Job drawing, mm, ordinate dimensions from the low corner. One solid piece. Round coordinates to 2 decimals unless told otherwise and drop trailing zeros. Loops run counter-clockwise (first coordinate to the right, second up) from the corner with the lowest first, then second, coordinate; pieces in that order, holes last. Notation, with made-up numbers: (82, 31) - (121, 31) arc R29 cw to (121, 56) - close; hole circle Ø5 at (75.25, 10). An arc over 180 degrees is marked (long way). One line per question, with ' | ' between items. Start each with the question number.
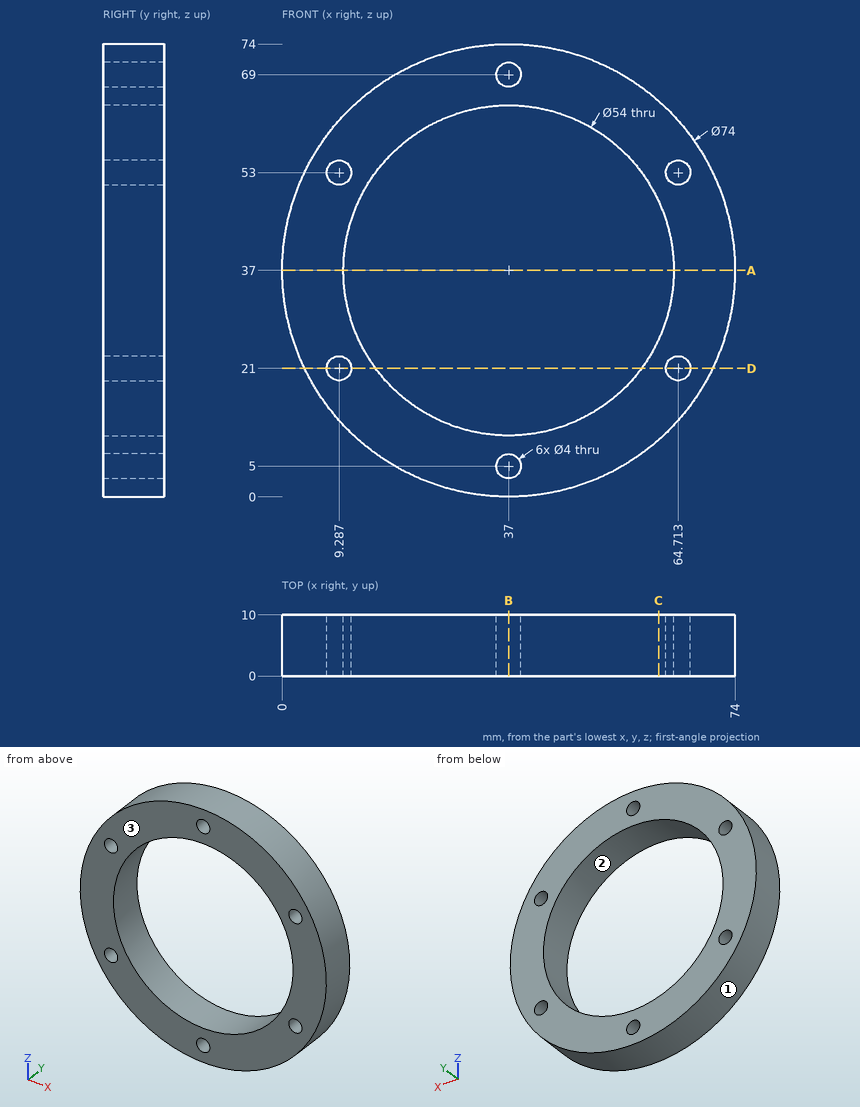
1) Wall check: line 1 (X direction, y = 7.5, z = 21); line 2 (X direction, y = 1.75, z = 19.5) (1 decimal); line 3 (X direction, y = 6, z = 37). Give the ranges that are in metal, low to high. Write a range as [from, to].
2) Saw through at B-B on x = 37. Write the cut outline in (y, z).
3) Saw through at A-A on z = 37. Write the cut outline in (x, y), and give its area (3 significant figures).
4) Saw through at D-D on z = 21. Write the cut outline in (x, y), and give its area (3 significant figures).
5) Drop flat-ended pins along their axis: pin 1 (3 mm diameter, centred on x = 8, y = 6.5, fed in from +Z); pin 2 (6 mm diameter, centred on y = 3, z = 65.5, fed in from -X); pin 3 (2 mm diameter, centred on y = 6, z = 19, fed in from -X). Give the stop position or say it passes through.
6) Two-plate mould, pull along X, no slides. Class the marked faces 1, 2 and 3: +X half, -X half, draft (parallel to the pull), parting line (faces both ways), or undercut.
7) Saw through at C-C on x = 61.5. Write the cut outline in (y, z), and give its area (3 significant figures).
Answer key:
1) line 1: [3.64, 7.29], [11.29, 15.25], [58.75, 62.71], [66.71, 70.36] | line 2: [4.4, 8], [10.6, 16.4], [57.6, 63.4], [66, 69.6] | line 3: [0, 10], [64, 74]
2) outline: (0, 0) - (10, 0) - (10, 3) - (0, 3) - close; (0, 7) - (10, 7) - (10, 10) - (0, 10) - close; (0, 64) - (10, 64) - (10, 67) - (0, 67) - close; (0, 71) - (10, 71) - (10, 74) - (0, 74) - close
3) outline: (0, 0) - (10, 0) - (10, 10) - (0, 10) - close; (64, 0) - (74, 0) - (74, 10) - (64, 10) - close | area: 200 mm²
4) outline: (3.64, 0) - (7.29, 0) - (7.29, 10) - (3.64, 10) - close; (11.29, 0) - (15.25, 0) - (15.25, 10) - (11.29, 10) - close; (58.75, 0) - (62.71, 0) - (62.71, 10) - (58.75, 10) - close; (66.71, 0) - (70.36, 0) - (70.36, 10) - (66.71, 10) - close | area: 152 mm²
5) pin 1: z = 61.75 | pin 2: x = 10.19 | pin 3: x = 4.14
6) face 1: parting line | face 2: undercut | face 3: draft
7) outline: (0, 9.27) - (10, 9.27) - (10, 25.65) - (0, 25.65) - close; (0, 48.35) - (10, 48.35) - (10, 64.73) - (0, 64.73) - close | area: 328 mm²
